Part model, mm, in its own coordinate system. Face numbers are marked on the shaded views. A direction names the side the tool comes from. Round coordinates to 2 decimals unless told otherwise and drop trailing zeros. Write each loop counter-clockwise with the first axis right and the second up, starting at its lowest first coordinate (ties: lowest second). Pieces come first, ordered by that corner, then holes. Notation, with made-up numbers: M -13,72.5 L 21,72.5 A7 cw 21,76.5 Z; hole C -14.5,51.25 d2. An arc over 180 degrees is marked long. Use a Markdown table: item, result. Add a question column.
1) Which spindle directions (+Z, -Z, +X, -X, +Y, -Y) get a long thin tool onto all of the face, cutting with end or side? Do the marked faces 1 and 2. Say none if no direction does.
2) Slice it at B-B on x = -24.25. Write the cut outline in (y, z) (3 decimals), plus the area to 3 significant figures.
3) Drop flat-ended pins along their axis: P1, Ø8, axis at y = -9, z = 7.5, coming from the -X side (3 decimals); P2, Ø8.5, axis at x = -22.225, z = 12.065, coming from the -Y side. Give the stop position or say it passes through.
4) Wall check: probe 1 along X at (y, z) = (-15, 14.75) (3 decimals); probe 2 along Y at (x, z) = (-15.25, 6) (3 decimals); probe 3 along Z at (x, y) = (-7.5, 1.25). Give the ranges that are in metal, low to high.
5) Two-plate mould, pull along Z, no slides. Class the marked faces 3, 4 and 5: released by +Z, released by -Z, zero draft, split by the parting line, or undercut.
6) Slice it at C-C on y = -17.75. Write the cut outline in (x, z) (3 decimals), plus the area to 3 significant figures.
7) Slice it at D-D on y = -3.5. Write the cut outline in (x, z) (3 decimals), plus the area to 3 significant figures.
8) Slice it at A-A on z = 11.5. Write the cut outline in (x, y) (3 decimals).
```python
from build123d import *

# Parameters (mm, degrees)
SKETCH1_W           = 28.575
SKETCH1_H           = 3.175
SKETCH1_W_2         = 3.175
SKETCH1_H_2         = 25.4
BOSS_EXTRUDE1_DEPTH = 19.05
SWITCH_MOUNT_REACH  = 5.175
SKETCH2_R           = 1.190625
SKETCH2_W           = 2.54
SKETCH2_H           = 0.254
BRACKET_MOUNT_REACH = 5.175
SKETCH3_R           = 3.175


with BuildPart() as part:
    # Sketch1 → Boss-Extrude1 (new body)
    with BuildSketch(Plane.XY):
        with Locations((-14.2875, 1.5875)):
            Rectangle(SKETCH1_W, SKETCH1_H)
        with Locations((-1.5875, -12.7)):
            Rectangle(SKETCH1_W_2, SKETCH1_H_2)
    extrude(amount=BOSS_EXTRUDE1_DEPTH)

    # Sketch2 → Switch Mount (cut, up to next)
    with BuildSketch(Plane.ZY.offset(3.175), mode=Mode.PRIVATE) as switch_mount_sk1:
        with Locations((4.9022, -8.636)):
            Circle(SKETCH2_R)
    switch_mount_tool1 = extrude(switch_mount_sk1.sketch, amount=-SWITCH_MOUNT_REACH, mode=Mode.PRIVATE) & part.part
    add(switch_mount_tool1.solids().sort_by_distance((-3.175, -8.636, 4.9022))[0], mode=Mode.SUBTRACT)
    # Sketch2 → Switch Mount (cut, up to next)
    with BuildSketch(Plane.ZY.offset(3.175), mode=Mode.PRIVATE) as switch_mount_sk2:
        with Locations((4.9022, -18.161)):
            Circle(SKETCH2_R)
    switch_mount_tool2 = extrude(switch_mount_sk2.sketch, amount=-SWITCH_MOUNT_REACH, mode=Mode.PRIVATE) & part.part
    add(switch_mount_tool2.solids().sort_by_distance((-3.175, -18.161, 4.9022))[0], mode=Mode.SUBTRACT)
    # Sketch2 → Switch Mount (cut, up to next)
    with BuildSketch(Plane.ZY.offset(3.175), mode=Mode.PRIVATE) as switch_mount_sk3:
        with Locations((1.27, -23.1902)):
            Rectangle(SKETCH2_W, SKETCH2_H)
    switch_mount_tool3 = extrude(switch_mount_sk3.sketch, amount=-SWITCH_MOUNT_REACH, mode=Mode.PRIVATE) & part.part
    add(switch_mount_tool3.solids().sort_by_distance((-3.175, -23.1902, 1.27))[0], mode=Mode.SUBTRACT)

    # Sketch3 → Bracket Mount (cut, up to next)
    with BuildSketch(Plane.XZ, mode=Mode.PRIVATE) as bracket_mount_sk1:
        with Locations((-9.525, 12.065)):
            Circle(SKETCH3_R)
    bracket_mount_tool1 = extrude(bracket_mount_sk1.sketch, amount=-BRACKET_MOUNT_REACH, mode=Mode.PRIVATE) & part.part
    add(bracket_mount_tool1.solids().sort_by_distance((-9.525, 0, 12.065))[0], mode=Mode.SUBTRACT)
    # Sketch3 → Bracket Mount (cut, up to next)
    with BuildSketch(Plane.XZ, mode=Mode.PRIVATE) as bracket_mount_sk2:
        with Locations((-22.225, 12.065)):
            Circle(SKETCH3_R)
    bracket_mount_tool2 = extrude(bracket_mount_sk2.sketch, amount=-BRACKET_MOUNT_REACH, mode=Mode.PRIVATE) & part.part
    add(bracket_mount_tool2.solids().sort_by_distance((-22.225, 0, 12.065))[0], mode=Mode.SUBTRACT)


solid = part.part
```
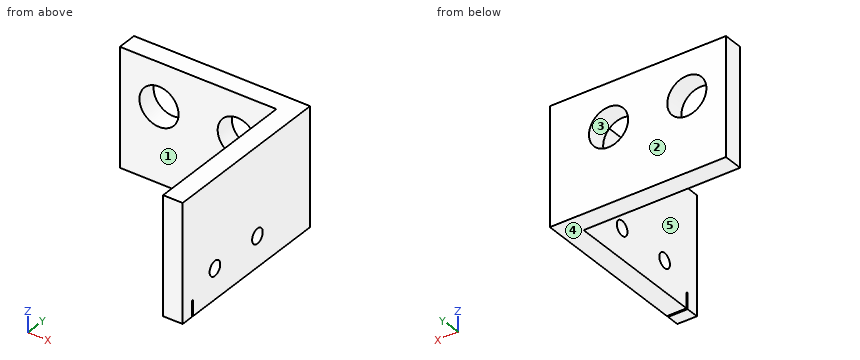
Entries:
| question | item | result |
|---|---|---|
| 1 | face 1 | +Z, -Z, -X, -Y |
| 1 | face 2 | +Z, -Z, +X, -X, +Y |
| 2 | outline | M 0,0 L 3.175,0 L 3.175,9.62 L 0,9.62 Z; M 0,14.51 L 3.175,14.51 L 3.175,19.05 L 0,19.05 Z |
| 2 | area | 45.0 mm^2 |
| 3 | P1 | stops at x = -3.175 |
| 3 | P2 | stops at y = 0 |
| 4 | probe 1 | x = -3.175 to 0 |
| 4 | probe 2 | y = 0 to 3.175 |
| 4 | probe 3 | z = 0 to 9.62, 14.51 to 19.05 |
| 5 | face 3 | undercut |
| 5 | face 4 | released by -Z |
| 5 | face 5 | zero draft |
| 6 | outline | M -3.175,0 L 0,0 L 0,3.785 L -3.175,3.785 Z; M -3.175,6.02 L 0,6.02 L 0,19.05 L -3.175,19.05 Z |
| 6 | area | 53.4 mm^2 |
| 7 | outline | M -3.175,0 L 0,0 L 0,19.05 L -3.175,19.05 Z |
| 7 | area | 60.5 mm^2 |
| 8 | outline | M -28.575,0 L -25.349,0 L -25.349,3.175 L -28.575,3.175 Z; M -19.101,0 L -12.649,0 L -12.649,3.175 L -19.101,3.175 Z; M -6.401,0 L -3.175,0 L -3.175,-25.4 L 0,-25.4 L 0,3.175 L -6.401,3.175 Z |
